Drawing for the job (mm, zero at the part's lowest x, y, z). A direction names the side the tool comes from. Give positions to 0.01 mm unless a question says otherwise; leave off trailing zeros. Order: outer loops, then holes, each group sorted by start corner. A loop starts at its lowest first (then second) coordinate and runs counter-clockwise, first axis right, second up. Notation, with made-up numbers: (-17.75, -15) - (35.25, -15) arc R18 ccw to (35.25, 2) - close; hole circle Ø9 at (-37.5, 30.5). An arc over 180 degrees is marked (long way). One line per item, written item: value.
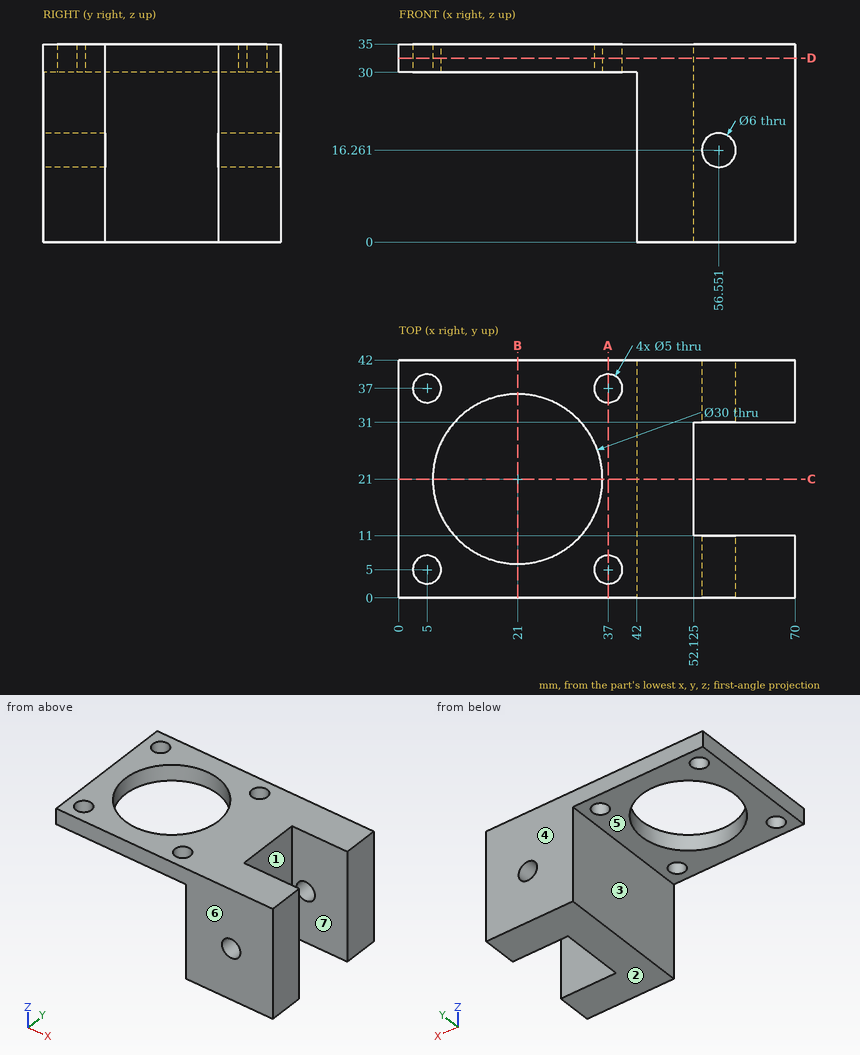
(1) Pin check, flat tips, straight feed: P1, Ø8, axis at x = 5, y = 37, coming from the -Z side; P2, Ø10, axis at y = 23, z = 12.5, coming from the +X side (3 decimals); P3, Ø9, axis at y = 20, z = 15, coming from the -X side; P4, Ø5.5, axis at x = 61.5, z = 10, coming from the -Y side. Stop position of each tip, or through.
Completed:
P1: z = 30
P2: x = 52.125
P3: x = 42
P4: y = 0
(2) 3-axis set-ups, long thin cutter, end or side, ignore diameter. For the marked faces 1, 2 and 3: which of +Z, -Z, +X, -X, +Y, -Y reach the whole face in a straight line?
Completed:
face 1: +Z, -Z, +X
face 2: -Z, +X, -X, +Y, -Y
face 3: -Z, -X, +Y, -Y
(3) Slice it at A-A, the plane x = 37. Give the cut face in (y, z).
Completed:
outline: (0, 30) - (2.5, 30) - (2.5, 35) - (0, 35) - close; (7.5, 30) - (34.5, 30) - (34.5, 35) - (7.5, 35) - close; (39.5, 30) - (42, 30) - (42, 35) - (39.5, 35) - close
(4) Slice it at D-D, the plane z = 32.5. Give the cut face in (x, y) (3 decimals).
Completed:
outline: (0, 0) - (70, 0) - (70, 11) - (52.125, 11) - (52.125, 31) - (70, 31) - (70, 42) - (0, 42) - close; hole circle Ø5 at (5, 5); hole circle Ø5 at (5, 37); hole circle Ø30 at (21, 21); hole circle Ø5 at (37, 5); hole circle Ø5 at (37, 37)
(5) Slice it at C-C, the plane y = 21. Give the cut face in (x, z) (3 decimals), and give its area (3 significant figures).
Completed:
outline: (0, 30) - (6, 30) - (6, 35) - (0, 35) - close; (36, 30) - (42, 30) - (42, 0) - (52.125, 0) - (52.125, 35) - (36, 35) - close
area: 414 mm²
(6) Drill centre lines: line 1 (Y direction, x = 37, z = 31); line 2 (Y direction, x = 53, z = 32); line 3 (X direction, y = 38.5, z = 19.5). Where is each one in solid material? Low to high.
Completed:
line 1: 0 to 2.5, 7.5 to 34.5, 39.5 to 42
line 2: 0 to 11, 31 to 42
line 3: 42 to 70
(7) Pull direction Y, two halves, no side cores. Call the marked faces 4, 5, 6 and 7: +Y half, -Y half, draft (parallel to the pull), parting line (faces both ways), or undercut.
Completed:
face 4: +Y half
face 5: draft
face 6: -Y half
face 7: undercut
(8) Slice it at B-B, the plane x = 21. Give the cut face in (y, z).
Completed:
outline: (0, 30) - (6, 30) - (6, 35) - (0, 35) - close; (36, 30) - (42, 30) - (42, 35) - (36, 35) - close
